Design review of the part built by this model. Coordinates are the model's own, in mm. Face numbers are marked on the shaded views. A direction names the side the tool comes from. Round coordinates to 2 decimals unless told otherwise and drop trailing zeros. Order: outer loops, then holes, each group sorted by start corner. A loop starts at its lowest first (then second) coordinate and runs counter-clockwise, first axis right, second up. Notation, with made-up numbers: (-19.5, 66.25) - (13.5, 66.25) arc R31 ccw to (13.5, 91.25) - close; hole circle Ø6 at (72, -15.75). An arc over 180 degrees is marked (long way). Use CSV: the item, a comma, the result in double quotes. Start each with the question number.
from build123d import *

# Parameters (mm, degrees)
F0_W     = 60
F0_H     = 140
F1_DEPTH = 0.5
F2_W     = 22
F2_H     = 70
F3_DEPTH = 0.5
F5_DEPTH = 0.2
F7_DEPTH = 0.2
F8_R     = 25
F9_R     = 5


with BuildPart() as f1:
    # F0 (on Front) → F1 (new body)
    with BuildSketch(Plane.XZ):
        Rectangle(F0_W, F0_H)
    extrude(amount=F1_DEPTH)

    # F2 (on face) → F3 (cut, through all)
    with BuildSketch(Plane.XZ.offset(0.5)):
        with Locations((0, -35)):
            Rectangle(F2_W, F2_H)
    extrude(amount=-F3_DEPTH, mode=Mode.SUBTRACT)

    # F4 (on face) → F5 (join)
    with BuildSketch(Plane.XZ.offset(0.5)):
        Polygon((-30, 70), (-30, -70), (-11, -70), (-11, 0), align=None)
    extrude(amount=F5_DEPTH)

    # F6 (on face) → F7 (join)
    with BuildSketch(Plane(origin=(0, 0, 0), x_dir=(-1, 0, 0), z_dir=(0, 1, 0))):
        Polygon((11, 0), (11, -70), (30, -70), (30, 70), align=None)
    extrude(amount=F7_DEPTH)

    # F8
    f8_edges = [f1.edges().sort_by_distance(p)[0] for p in [
        (30, -0.25, 70),
    ]]
    fillet(f8_edges, radius=F8_R)

    # F9
    f9_edges = [f1.edges().sort_by_distance(p)[0] for p in [
        (-30, -0.25, -70),
        (-11, -0.25, -70),
        (11, -0.25, -70),
        (30, -0.25, -70),
    ]]
    fillet(f9_edges, radius=F9_R)


solid = f1.part
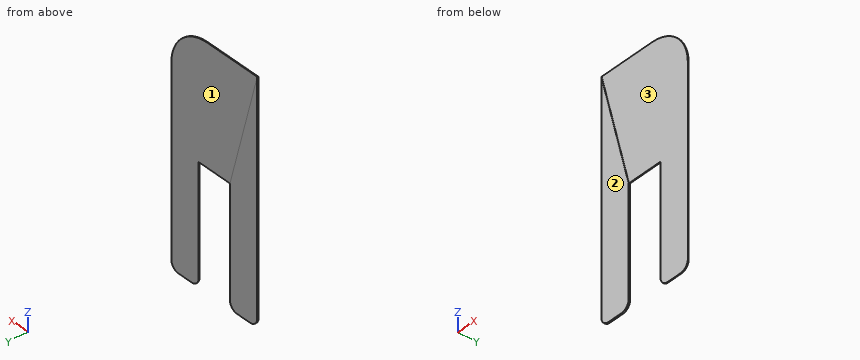
Q1. Take a section at D-D (z = 41). State the section outline as (x, y) points.
Q2. Take a section at B-B (y = -0.25). State the section outline as (x, z) points.
Q3. Tool access review of the marked faces 1, 2 and 3: name each direction out of +Z, -Z, +X, -X, +Y, -Y from which nothing blocks a thin tool from reaching the whole face with its end or side.
Q4. Take a section at A-A (z = -23). State the section outline as (x, y) points.
Q5. For L1, parallel to X at y = -0.05, z = -29.5; L2, parallel to X at y = 0.05, z = -12.5; L3, parallel to Y at x = 11, z = 46, list the stretches that pass through material, from the lowest coordinate up. Write a range as [from, to].
Q6. Take a section at C-C (x = -20.5). State the section outline as (y, z) points, plus the area to 3 significant figures.
Findings below:
1,outline,"(-30, -0.7) - (-22.13, -0.7) - (-22.13, -0.5) - (30, -0.5) - (30, 0) - (-22.13, 0) - (-22.13, 0.2) - (-30, 0.2) - close"
2,outline,"(-30, -65) arc R5 ccw to (-25, -70) - (-16, -70) arc R5 ccw to (-11, -65) - (-11, 0) - (11, 0) - (11, -65) arc R5 ccw to (16, -70) - (25, -70) arc R5 ccw to (30, -65) - (30, 45) arc R25 ccw to (5, 70) - (-30, 70) - close"
3,face 1,"+Z, +X, +Y"
3,face 2,"+Z, -Z, +X, -X, -Y"
3,face 3,"+Z, +X, -Y"
4,outline,"(-30, -0.7) - (-11, -0.7) - (-11, 0.2) - (-30, 0.2) - close; (11, -0.5) - (30, -0.5) - (30, 0) - (11, 0) - close"
5,L1,"x = [-30, -11], [11, 30]"
5,L2,"x = [-30, -11]"
5,L3,"y = [-0.5, 0]"
6,outline,"(-0.7, -70) - (0.2, -70) - (0.2, 35) - (0, 35) - (0, 70) - (-0.5, 70) - (-0.5, 35) - (-0.7, 35) - close"
6,area,"112 mm^2"
